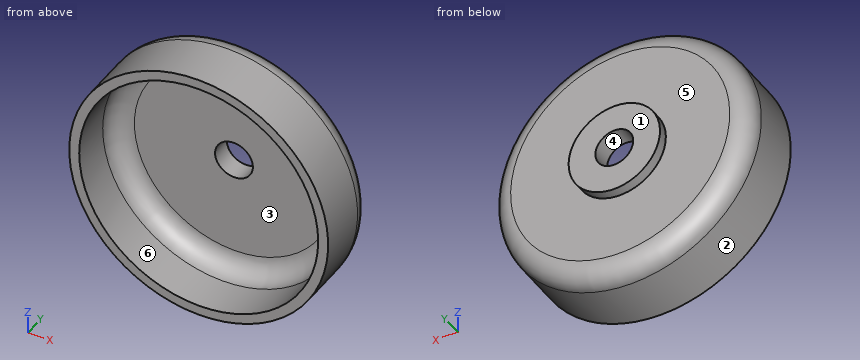
```python
from build123d import *

# Parameters (mm, degrees)
SKETCH1_R           = 65
BOSS_EXTRUDE1_DEPTH = 35
SKETCH2_R           = 22.945
BOSS_EXTRUDE2_DEPTH = 5
SKETCH3_R           = 9.5
CUT_EXTRUDE1_DEPTH  = 99
SKETCH4_R           = 60
CUT_EXTRUDE2_DEPTH  = 30
FILLET1_R           = 10
FILLET2_R           = 10


with BuildPart() as part:
    # Sketch1 → Boss-Extrude1 (new body)
    with BuildSketch(Plane(origin=(0, 0, 0), x_dir=(1, 0, 0), z_dir=(0, 1, 0))):
        with Locations(Location((0, 0, 0), (0, 0, 270))):
            Circle(SKETCH1_R)
    extrude(amount=BOSS_EXTRUDE1_DEPTH)

    # Sketch2 → Boss-Extrude2 (add)
    with BuildSketch(Plane(origin=(0, 35, 0), x_dir=(1, 0, 0), z_dir=(0, 1, 0))):
        with Locations(Location((0, 0, 0), (0, 0, 270))):
            Circle(SKETCH2_R)
    extrude(amount=BOSS_EXTRUDE2_DEPTH)

    # Sketch3 → Cut-Extrude1 (cut)
    with BuildSketch(Plane(origin=(0, 40, 0), x_dir=(1, 0, 0), z_dir=(0, 1, 0))):
        with Locations(Location((0, 0, 0), (0, 0, 270))):
            Circle(SKETCH3_R)
    extrude(amount=-CUT_EXTRUDE1_DEPTH, mode=Mode.SUBTRACT)

    # Sketch4 → Cut-Extrude2 (cut)
    with BuildSketch(Plane.XZ):
        with Locations(Location((0, 0, 0), (0, 0, 270))):
            Circle(SKETCH4_R)
    extrude(amount=-CUT_EXTRUDE2_DEPTH, mode=Mode.SUBTRACT)

    # Fillet1
    fillet1_edges = [part.edges().sort_by_distance(p)[0] for p in [
        (0, 35, -65),
    ]]
    fillet(fillet1_edges, radius=FILLET1_R)

    # Fillet2
    fillet2_edges = [part.edges().sort_by_distance(p)[0] for p in [
        (0, 30, 60),
    ]]
    fillet(fillet2_edges, radius=FILLET2_R)


solid = part.part
```
Read the model definition and answer for the solid it produces. Units are mm, in the model's axes. Face numbers are marked on the shaded views. A direction names the side the tool comes from. Round coordinates to 2 decimals unless told otherwise and drop trailing zeros. Write each loop counter-clockwise with the first axis right and the second up, starting at its lowest first coordinate (ties: lowest second). Pieces come first, ordered by that corner, then holes. Notation, with made-up numbers: M -8,62 L 41,62 A17 ccw 41,89 Z; hole C 13,63.25 d1. An arc over 180 degrees is marked long. One line per item, written item: value.
Q1. Flat-ended cylindrical pins translate along their axes: pin 1 Ø3 at (x, z) = (41.5, 44) entering from +Y; pin 2 Ø6 at (x, z) = (49.5, 12) entering from +Y; pin 3 Ø5 at (y, z) = (27.5, -5) entering from -X. Find the tip coordinate at first contact, or state that the pin passes through.
Data:
pin 1: y = 34.17
pin 2: y = 35
pin 3: x = -64.89
Q2. Find section C-C on y = 37.5. Write down the section's boundary in (x, z) (3 decimals), plus the area to 3 significant figures.
Data:
outline: C 0,0 d45.89; hole C 0,0 d19
area: 1,370 mm2
Q3. Straight lines are drawn through the part: line 1 (X direction, y = 11, z = 0); line 2 (Y direction, x = -28, z = 30); line 3 (X direction, y = 33, z = 0). For each, find the intervals that lie inside material, in ascending order. Write a range as [from, to].
Data:
line 1: [-65, -60], [60, 65]
line 2: [30, 35]
line 3: [-61, -9.5], [9.5, 61]
Q4. For a pull along Z with two mould halves and no side action, classify the marked faces 1, 2, 3 and 4 as +Z half, -Z half, draft (parallel to the pull), parting line (faces both ways), or undercut.
Data:
face 1: draft
face 2: parting line
face 3: undercut
face 4: undercut
Q5. Find section D-D on y = 13. Write down the section's boundary in (x, z).
Data:
outline: C 0,0 d130; hole C 0,0 d120
Q6. Find section B-B on z = 0. Write down the section's boundary in (x, y) (3 decimals), plus the area to 3 significant figures.
Data:
outline: M -65,0 L -60,0 L -60,20 A10 cw -50,30 L -9.5,30 L -9.5,40 L -22.945,40 L -22.945,35 L -55,35 A10 ccw -65,25 Z; M 9.5,30 L 50,30 A10 cw 60,20 L 60,0 L 65,0 L 65,25 A10 ccw 55,35 L 22.945,35 L 22.945,40 L 9.5,40 Z
area: 989 mm2
Q7. Which of the six approach directions +Z, -Z, +X, -X, +Y, -Y give full straight-line access (tool end or side, diameter ignored) to the marked faces 5 and 6?
Data:
face 5: +Y
face 6: -Y
Q8. Find section A-A on x = 0. Write down the section's boundary in (y, z) (3 decimals), plus the area to 3 significant figures.
Data:
outline: M 0,-65 L 25,-65 A10 ccw 35,-55 L 35,-22.945 L 40,-22.945 L 40,-9.5 L 30,-9.5 L 30,-50 A10 cw 20,-60 L 0,-60 Z; M 0,60 L 20,60 A10 cw 30,50 L 30,9.5 L 40,9.5 L 40,22.945 L 35,22.945 L 35,55 A10 ccw 25,65 L 0,65 Z
area: 989 mm2
